Build history of the part. All positions in model axes, mm. A direction names the side the tool comes from. Round coordinates to 2 decimals unless told otherwise and drop trailing zeros. Write each loop counter-clockwise with the first axis right and the second up, starting at its lowest first coordinate (ties: lowest second). Pieces come first, ordered by that corner, then holes. Notation, with made-up numbers: (-39.75, 33.25) -> (-21.75, 33.25) arc R26 ccw to (-21.75, 61.25) -> close; hole circle Ø9 at (-11, -20.75). An arc over 180 degrees is marked (long way). Answer in a Markdown table with one row per item. Add a question column.
from build123d import *

# Parameters (mm, degrees)
SZKIC1_R                    = 55
SZKIC1_R_2                  = 5
SZKIC1_R_3                  = 4.25
DODANIE_WYCI_GNI_CIE1_DEPTH = 30
WYTNIJ_WYCI_GNI_CIE1_DEPTH  = 30
ZAOKR_GLENIE1_R             = 10


with BuildPart() as part:
    # Szkic1 → Dodanie-wyciągnięcie1 (new body)
    with BuildSketch(Plane.XY):
        with BuildLine():
            Line((-38, 260), (38, 260))
            ThreePointArc((38, 260), (50.853486978, 256.267902519), (59.709435091, 246.232322709))
            Line((59.709435091, 246.232322709), (90.008216267, 181.948831851))
            ThreePointArc((90.008216267, 181.948831851), (91.483769879, 171.062118236), (86.44222441, 161.300939461))
            ThreePointArc((86.44222441, 161.300939461), (73.499977081, 129.92645546), (86.44222441, 98.551971459))
            ThreePointArc((86.44222441, 98.551971459), (91.483769879, 88.790792684), (90.008216267, 77.904079069))
            Line((90.008216267, 77.904079069), (59.766160901, 13.740940677))
            ThreePointArc((59.766160901, 13.740940677), (50.88106069, 3.705595357), (38, 0))
            Line((38, 0), (0, 0))
            Line((0, 0), (-38, 0))
            ThreePointArc((-38, 0), (-50.88106069, 3.705595357), (-59.766160901, 13.740940677))
            Line((-59.766160901, 13.740940677), (-90.008216267, 77.904079069))
            ThreePointArc((-90.008216267, 77.904079069), (-91.483769879, 88.790792684), (-86.44222441, 98.551971459))
            ThreePointArc((-86.44222441, 98.551971459), (-73.499977081, 129.92645546), (-86.44222441, 161.300939461))
            ThreePointArc((-86.44222441, 161.300939461), (-91.483769879, 171.062118236), (-90.008216267, 181.948831851))
            Line((-90.008216267, 181.948831851), (-59.709435091, 246.232322709))
            ThreePointArc((-59.709435091, 246.232322709), (-50.853486978, 256.267902519), (-38, 260))
        make_face()
        with Locations((0, 130)):
            Circle(SZKIC1_R, mode=Mode.SUBTRACT)
        with Locations((-73, 87)):
            Circle(SZKIC1_R_2, mode=Mode.SUBTRACT)
        with Locations(Location((-73, 173, 0), (0, 0, 180))):
            Circle(SZKIC1_R_2, mode=Mode.SUBTRACT)
        with Locations((25, 230)):
            Circle(SZKIC1_R_3, mode=Mode.SUBTRACT)
        with Locations((-24.992384758, 229.127379678)):
            Circle(SZKIC1_R_3, mode=Mode.SUBTRACT)
        with Locations((-25, 30)):
            Circle(SZKIC1_R_3, mode=Mode.SUBTRACT)
        with Locations((24.931476738, 27.383202188)):
            Circle(SZKIC1_R_3, mode=Mode.SUBTRACT)
    extrude(amount=DODANIE_WYCI_GNI_CIE1_DEPTH)

    # Szkic4 → Wytnij-wyciągnięcie1 (cut)
    with BuildSketch(Plane(origin=(-86.44222441, 98.551971459, 0), x_dir=(-1, 0, 0), z_dir=(0, 0, -1))):
        Polygon((-52.536909819, -48.057816777), (-50.443471569, -88.002998167), (-120.347539002, -91.666515104), (-122.440977251, -51.721333714), align=None)
    extrude(amount=-WYTNIJ_WYCI_GNI_CIE1_DEPTH, mode=Mode.SUBTRACT)

    # Zaokrąglenie1
    zaokr_glenie1_edges = [part.edges().sort_by_distance(p)[0] for p in [
        (35.998752841, 46.830637745, 15),
        (-33.905314592, 50.494154682, 15),
        (-35.998752841, 10.548973291, 15),
        (33.905314592, 6.885456354, 15),
    ]]
    fillet(zaokr_glenie1_edges, radius=ZAOKR_GLENIE1_R)


solid = part.part
(1) Which spindle directions (+Z, -Z, +X, -X, +Y, -Y) get a long thin tool onto all of the face, cutting with end or side? Do faces 1 (the face through (-74.675, 45.373, 14.79)), 2 (the face through (1.396, 48.644, 14.79)). Say none if no direction does.
(2) Probe line 1 along X through (y, z) = (169.5, 13); line 2 along Y through (x, z) = (28.5, 5); line 3 along Y through (x, z) = (17, 25.75). List the from-to ranges inside material, lowest first.
(3) Drop flat-ended pins along their axis: P1, Ø6, axis at x = 58, z = 19.5, coming from the +Y side; P2, Ø10, axis at y = 51, z = 25.5, coming from the +X side; P3, Ø8, axis at y = 231.5, z = 18.5, coming from the +X side. Give the stop position or say it passes through.
(4) Saw through at A-A (y = 173). List the corners of the cut face in (x, z).
(5) Saw through at C-C (y = 119). List the corners of the cut face in (x, z).
(6) Mould opens along Y. For faces 3 (the face through (-75.07, 213.64, 14.79)), 4 (the face through (1, 0, 15)), 5 (the face through (-34.945, 30.661, 14.79)), 6 (the face through (34.945, 26.718, 14.79)) say: pulls with the +Y half, pulls with the -Y half, needs draft (parallel to the pull), parting line crosses it, or undercut.
(7) Saw through at B-B (x = 48.5). List the corners of the cut face in (y, z).
(8) Saw through at D-D (x = 0). List the corners of the cut face in (y, z).
Answer sheet:
| question | item | result |
|---|---|---|
| 1 | face 1 | +Z, -Z, -X, -Y |
| 1 | face 2 | +Z, -Z |
| 2 | line 1 | x = -91.14 to -76.57, -69.43 to -38.27, 38.27 to 91.14 |
| 2 | line 2 | y = 0 to 8.26, 46.9 to 82.96, 177.04 to 227.59, 232.41 to 260 |
| 2 | line 3 | y = 0 to 7.77, 47.83 to 77.69, 182.31 to 260 |
| 3 | P1 | stops at y = 252.94 |
| 3 | P2 | stops at x = 79.68 |
| 3 | P3 | stops at x = 68.54 |
| 4 | outline | (-91.71, 0) -> (-78, 0) -> (-78, 30) -> (-91.71, 30) -> close; (-68, 0) -> (-34.29, 0) -> (-34.29, 30) -> (-68, 30) -> close; (34.29, 0) -> (91.71, 0) -> (91.71, 30) -> (34.29, 30) -> close |
| 5 | outline | (-74.86, 0) -> (-53.89, 0) -> (-53.89, 30) -> (-74.86, 30) -> close; (53.89, 0) -> (74.86, 0) -> (74.86, 30) -> (53.89, 30) -> close |
| 6 | face 3 | pulls with the +Y half |
| 6 | face 4 | pulls with the -Y half |
| 6 | face 5 | undercut |
| 6 | face 6 | undercut |
| 7 | outline | (2.39, 0) -> (104.06, 0) -> (104.06, 30) -> (2.39, 30) -> close; (155.94, 0) -> (257.58, 0) -> (257.58, 30) -> (155.94, 30) -> close |
| 8 | outline | (0, 0) -> (8.66, 0) -> (8.66, 30) -> (0, 30) -> close; (48.72, 0) -> (75, 0) -> (75, 30) -> (48.72, 30) -> close; (185, 0) -> (260, 0) -> (260, 30) -> (185, 30) -> close |
